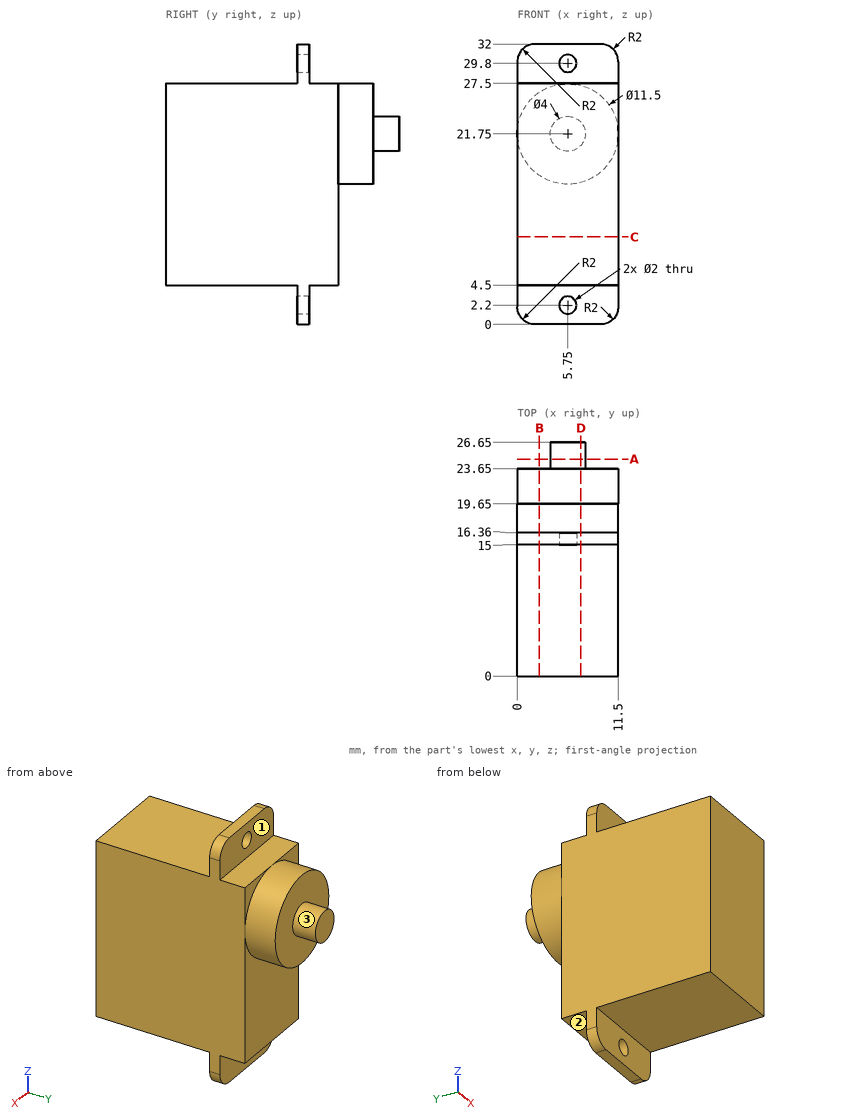
Here's the drawing with two shaded views (mm, measured from the low corner). I have some questions. A direction names the side the tool comes from. Coordinates: 2 decimals unless noted, no trailing zeros. Order: outer loops, then holes, each group sorted by start corner. A loop starts at its lowest first (then second) coordinate and runs counter-clockwise, first axis right, second up. Notation, with made-up numbers: (-20.75, 59) -> (-5.75, 59) arc R6 cw to (-5.75, 68) -> close; hole circle Ø8 at (52, -22). An arc over 180 degrees is marked (long way). Write each question's results on one line, items separated by ' | '.
Item 1: I want a section at B-B, the plane x = 2.5. Write out the boundary of the cut face in (y, z).
Results are:
outline: (0, 4.5) -> (15, 4.5) -> (15, 0) -> (16.36, 0) -> (16.36, 4.5) -> (19.65, 4.5) -> (19.65, 17.01) -> (23.65, 17.01) -> (23.65, 26.49) -> (19.65, 26.49) -> (19.65, 27.5) -> (16.36, 27.5) -> (16.36, 32) -> (15, 32) -> (15, 27.5) -> (0, 27.5) -> close
Item 2: I want a section at D-D, the plane x = 7.25. Write out the boundary of the cut face in (y, z), then the cut area to 3 significant figures.
Results are:
outline: (0, 4.5) -> (15, 4.5) -> (15, 0) -> (16.36, 0) -> (16.36, 4.5) -> (19.65, 4.5) -> (19.65, 16.2) -> (23.65, 16.2) -> (23.65, 20.43) -> (26.65, 20.43) -> (26.65, 23.07) -> (23.65, 23.07) -> (23.65, 27.3) -> (19.65, 27.3) -> (19.65, 27.5) -> (16.36, 27.5) -> (16.36, 32) -> (15, 32) -> (15, 27.5) -> (0, 27.5) -> close | area: 517 mm²
Item 3: If I drill on line 1 along X through (y, z) = (15.75, 29.8); line 2 along Y through (x, z) = (3.25, 22.5); line 3 along Z through (x, y) = (5.25, 6), over which ranges is the centre line in solid material (lowest first)?
Results are:
line 1: 0 to 4.75, 6.75 to 11.5 | line 2: 0 to 23.65 | line 3: 4.5 to 27.5
Item 4: Which directions (+Z, -Z, +X, -X, +Y, -Y) give clear straight access to the entire face, cutting with the end or side of a thin tool? Please do the marked faces 1, 2 and 3.
Results are:
face 1: +Z, +X, -X, +Y | face 2: -Z, +X, -X, +Y | face 3: +Y
Item 5: I want a section at A-A, the plane y = 24.75. Write out the boundary of the cut face in (x, z), then the cut area to 3 significant figures.
Results are:
outline: circle Ø4 at (5.75, 21.75) | area: 12.6 mm²
Item 6: I want a section at C-C, the plane z = 10. Write out the boundary of the cut face in (x, y), then the cut area to 3 significant figures.
Results are:
outline: (0, 0) -> (11.5, 0) -> (11.5, 19.65) -> (0, 19.65) -> close | area: 226 mm²
Item 7: I'm going to push flat-ended pins straight in: pin 1 Ø3.5 at (x, z) = (6, 1.5) entering from -Y; pin 2 Ø3.5 at (x, z) = (6, 29.5) entering from +Y; pin 3 Ø5 at (x, y) = (5.5, 14) entering from +Z; pin 4 Ø1 at (x, y) = (9, 14) entering from -Z. Where does each tip first touch, or does it pass through?
Results are:
pin 1: y = 15 | pin 2: y = 16.36 | pin 3: z = 32 | pin 4: z = 4.5
